The listing builds one solid part. Answer for the finished solid, in the listing's coordinates (mm). Face numbers are marked on the shaded views. A direction names the side the tool comes from. Coordinates: 2 decimals unless noted, no trailing zeros. Write each loop counter-clockwise with the first axis right and the second up, starting at its lowest first coordinate (ties: lowest second). Pieces come first, ordered by that corner, then holes. Notation, with made-up numbers: M 34,-21 L 83,-21 A36 ccw 83,17 Z; hole C -4.5,-23.75 d9. An arc over 180 degrees is marked long. Put each result on its own line as item: value. Start each with the question number.
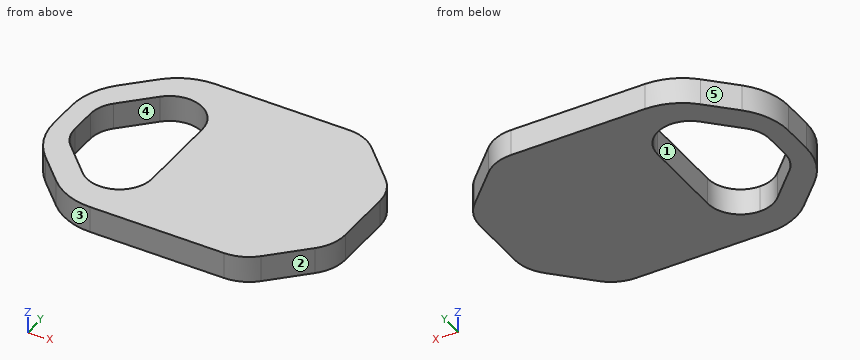
```python
from build123d import *

# Parameters (mm, degrees)
F1_DEPTH = 6.35


# Not quite as in the source:
# - a feature names something its author has since deleted; it is built from what else it names


with BuildPart() as f1:
    # F0 (on Top) → F1 (new body)
    with BuildSketch(Plane.XY):
        with BuildLine():
            ThreePointArc((69.4316146906, -39.8903370424), (71.634025844, -36.5941958184), (72.4074097937, -32.7061321456))
            Line((72.4074097937, -32.7061321456), (72.4074097937, -18.516951733))
            ThreePointArc((72.4074097937, -18.516951733), (71.634025844, -14.6288880601), (69.4316146906, -11.3327468361))
            Line((69.4316146906, -11.3327468361), (61.2862048969, -3.1873370424))
            ThreePointArc((61.2862048969, -3.1873370424), (57.9900636728, -0.9849258889), (54.102, -0.2115419393))
            Line((54.102, -0.2115419393), (21.9140133571, -0.2115419393))
            ThreePointArc((21.9140133571, -0.2115419393), (16.1111416714, -1.3595484607), (11.1825133635, -4.6306127791))
            Line((11.1825133635, -4.6306127791), (4.9301931337, -10.8312609409))
            ThreePointArc((4.9301931337, -10.8312609409), (1.4826892564, -15.9562170355), (0.2714097937, -22.0128877397))
            Line((0.2714097937, -22.0128877397), (0.2714097937, -29.2101961388))
            ThreePointArc((0.2714097937, -29.2101961388), (1.4826892564, -35.266866843), (4.9301931337, -40.3918229376))
            Line((4.9301931337, -40.3918229376), (11.1825133635, -46.5924710994))
            ThreePointArc((11.1825133635, -46.5924710994), (16.1111416714, -49.8635354178), (21.9140133571, -51.0115419393))
            Line((21.9140133571, -51.0115419393), (54.102, -51.0115419393))
            ThreePointArc((54.102, -51.0115419393), (57.9900636728, -50.2381579896), (61.2862048969, -48.0357468361))
            Line((61.2862048969, -48.0357468361), (69.4316146906, -39.8903370424))
        make_face()
        with BuildLine():
            Line((27.8558097937, -15.4515419393), (27.8558097937, -35.7715419393))
            ThreePointArc((27.8558097937, -35.7715419393), (25.5495685888, -41.3393007343), (19.9818097937, -43.6455419393))
            ThreePointArc((19.9818097937, -43.6455419393), (16.9685604473, -43.0461693783), (14.4140509986, -41.3393007343))
            Line((14.4140509986, -41.3393007343), (7.4036509986, -34.3289007343))
            ThreePointArc((7.4036509986, -34.3289007343), (5.6967823547, -31.7743912857), (5.0974097937, -28.7611419393))
            Line((5.0974097937, -28.7611419393), (5.0974097937, -22.4619419393))
            ThreePointArc((5.0974097937, -22.4619419393), (5.6967823547, -19.4486925928), (7.4036509986, -16.8941831442))
            Line((7.4036509986, -16.8941831442), (14.4140509986, -9.8837831442))
            ThreePointArc((14.4140509986, -9.8837831442), (22.9950591402, -8.1769145003), (27.8558097937, -15.4515419393))
        make_face(mode=Mode.SUBTRACT)
    extrude(amount=F1_DEPTH)


solid = f1.part
```
1) Given pin 1 Ø1.5 at (x, z) = (8, 1) entering from -Y; pin 2 Ø1 at (x, y) = (63.5, -14) entering from -Z; pin 3 Ø1 at (y, z) = (-13, 4) entering from -X; pin 4 Ø3 at (y, z) = (-45.5, 1) entering from -X, each flat-ended and moving along its own axis, determine where each tip first touches the part or whether it passes through.
2) Determine the mould class of the marked faces 1, 2 and 3 for opening direction X: +X half, -X half, draft (parallel to the pull), parting line (faces both ways), or undercut.
3) A cutting plane is placed at A-A on z = 1. Write down the section's boundary in (x, y).
4) A cutting plane is placed at C-C on x = 17. Write down the section's boundary in (y, z).
5) For the marked faces 4 and 5, determine the directions among +Z, -Z, +X, -X, +Y, -Y from which every point of the face is accessible in a straight line to the end or side of a thin tool.
6) A cutting plane is placed at B-B on y = -26.5. Write down the section's boundary in (x, z), then the cut area to 3 significant figures.
7) Straight lines are drawn through the part: probe 1 along X at (y, z) = (-29, 3.25); probe 2 along Y at (x, z) = (11, 4); probe 3 along X at (y, z) = (-39, 2.5). For each, find the intervals that lie inside material, in ascending order.
Answers follow:
1. pin 1: stops at y = -44.18
1. pin 2: stops at z = 0
1. pin 3: stops at x = 2.77
1. pin 4: stops at x = 8.57
2. face 1: undercut
2. face 2: +X half
2. face 3: -X half
3. outline: M 0.27,-29.21 A15.75 ccw 4.93,-40.39 L 11.18,-46.59 A15.24 ccw 21.91,-51.01 L 54.1,-51.01 A10.16 ccw 61.29,-48.04 L 69.43,-39.89 A10.16 ccw 72.41,-32.71 L 72.41,-18.52 A10.16 ccw 69.43,-11.33 L 61.29,-3.19 A10.16 ccw 54.1,-0.21 L 21.91,-0.21 A15.24 ccw 11.18,-4.63 L 4.93,-10.83 A15.75 ccw 0.27,-22.01 Z; hole M 5.1,-28.76 A7.87 ccw 7.4,-34.33 L 14.41,-41.34 A7.87 ccw 27.86,-35.77 L 27.86,-15.45 A7.87 ccw 14.41,-9.88 L 7.4,-16.89 A7.87 ccw 5.1,-22.46 Z
4. outline: M -50.2,0 L -43.06,0 L -43.06,6.35 L -50.2,6.35 Z; M -8.16,0 L -1.03,0 L -1.03,6.35 L -8.16,6.35 Z
5. face 4: +Z, -Z
5. face 5: +Z, -Z, -X, +Y
6. outline: M 0.27,0 L 5.1,0 L 5.1,6.35 L 0.27,6.35 Z; M 27.86,0 L 72.41,0 L 72.41,6.35 L 27.86,6.35 Z
6. area: 314 mm²
7. probe 1: x = 0.27 to 5.1, 27.86 to 72.41
7. probe 2: y = -46.41 to -37.93, -13.3 to -4.81
7. probe 3: x = 3.68 to 12.07, 27.16 to 70.22
